Geometry check sheet. Reference: the model listing, model coordinates, mm. A direction names the side the tool comes from. Give positions to 0.01 mm unless a question says otherwise; leave off trailing zeros. Write each loop counter-clockwise with the first axis right and the second up, starting at its lowest first coordinate (ties: lowest second). Pieces come first, ordered by that corner, then holes. Notation, with made-up numbers: (12, 6) - (16, 6) arc R6 cw to (16, 15) - close; hole circle Ø3 at (20.5, -22.5). An arc over 180 degrees is marked (long way). Write item = value, one per line. Start each with the question number.
(1) Access from +Z, -Z, +X, -X, +Y, -Y to the whole of each face (thin tool, end or side, straight path). Record for faces 4 (the cylindrical face through (23.059, 0.513, 5.07)), 5 (the flat face through (21, 3, 3)), 6 (the cylindrical face through (18.541, 3.487, 5.07)).
(2) Section check B-B, the plane x = 17. Enter the section's corners in (y, z), plus the area to 3 significant figures.
(3) Depth check by flat-ended pin: pin 1 Ø1.5 at (y, z) = (3.5, 2) entering from +X; pin 2 Ø1.2 at (x, y) = (15.5, 2.5) entering from +Z; pin 3 Ø1 at (x, z) = (41.5, 2.5) entering from -Y. Enter the tip coordinate at first touch or a pass-through.
(4) Draft check along Y on faces 1 (the flat face through (57, 3, 3)), 2 (the cylindrical face through (68.059, 0.513, 3.221)), 3 (the flat face through (61, 2, 0)). Enter one of: pulls with the +Y half, pulls with the -Y half, needs draft (parallel to the pull), parting line crosses it, or undercut.
(5) Section check A-A, the plane z = 1. Give the number of separate pieces and of enclosed holes in the cut face, plus the area to 4 significant figures.
(6) Thickness scan on L1, parallel to Y at x = 12, z = 0.5; L2, parallel to Z at x = 36, y = 3.2; L3, parallel to X at y = 3.65, z = -3. Record the ranges inside material, lowest first.
```python
from build123d import *

# Parameters (mm, degrees)
SKETCH008_W     = 68.6
SKETCH008_H     = 4
PAD_DEPTH       = 3.75
SKETCH_W        = 5.6
SKETCH_H        = 4
PAD001_DEPTH    = 10
SKETCH001_W     = 5.6
SKETCH001_H     = 4
PAD002_DEPTH    = 10
SKETCH002_W     = 5.6
SKETCH002_H     = 4
PAD003_DEPTH    = 10
SKETCH003_W     = 5.6
SKETCH003_H     = 4
PAD004_DEPTH    = 10
SKETCH004_W     = 5.6
SKETCH004_H     = 4
PAD005_DEPTH    = 10
SKETCH005_W     = 5.6
SKETCH005_H     = 4
PAD006_DEPTH    = 10
SKETCH006_W     = 5.6
SKETCH006_H     = 4
PAD007_DEPTH    = 10
SKETCH007_W     = 5.6
SKETCH007_H     = 4
PAD008_DEPTH    = 10
SKETCH009_W     = 3.6
SKETCH009_H     = 2
POCKET_DEPTH    = 13.75
SKETCH010_W     = 3.6
SKETCH010_H     = 2
POCKET001_DEPTH = 13.75
SKETCH011_W     = 3.6
SKETCH011_H     = 2
POCKET002_DEPTH = 13.75
SKETCH012_W     = 3.6
SKETCH012_H     = 2
POCKET003_DEPTH = 13.75
SKETCH013_W     = 3.6
SKETCH013_H     = 2
POCKET004_DEPTH = 13.75
SKETCH014_W     = 3.6
SKETCH014_H     = 2
POCKET005_DEPTH = 13.75
SKETCH015_W     = 3.6
SKETCH015_H     = 2
POCKET006_DEPTH = 13.75
SKETCH016_W     = 3.6
SKETCH016_H     = 2
POCKET007_DEPTH = 13.75
FILLET_R        = 1.8


with BuildPart() as part:
    # Sketch008 → Pad (new body)
    with BuildSketch(Plane.XY):
        with Locations((34.3, 2)):
            Rectangle(SKETCH008_W, SKETCH008_H)
    extrude(amount=-PAD_DEPTH)

    # Sketch → Pad001 (join)
    with BuildSketch(Plane.XY):
        with Locations((2.8, 2)):
            Rectangle(SKETCH_W, SKETCH_H)
    extrude(amount=PAD001_DEPTH)

    # Sketch001 → Pad002 (join)
    with BuildSketch(Plane.XY):
        with Locations((11.8, 2)):
            Rectangle(SKETCH001_W, SKETCH001_H)
    extrude(amount=PAD002_DEPTH)

    # Sketch002 → Pad003 (join)
    with BuildSketch(Plane.XY):
        with Locations((20.8, 2)):
            Rectangle(SKETCH002_W, SKETCH002_H)
    extrude(amount=PAD003_DEPTH)

    # Sketch003 → Pad004 (join)
    with BuildSketch(Plane.XY):
        with Locations((29.8, 2)):
            Rectangle(SKETCH003_W, SKETCH003_H)
    extrude(amount=PAD004_DEPTH)

    # Sketch004 → Pad005 (join)
    with BuildSketch(Plane.XY):
        with Locations((38.8, 2)):
            Rectangle(SKETCH004_W, SKETCH004_H)
    extrude(amount=PAD005_DEPTH)

    # Sketch005 → Pad006 (join)
    with BuildSketch(Plane.XY):
        with Locations((47.8, 2)):
            Rectangle(SKETCH005_W, SKETCH005_H)
    extrude(amount=PAD006_DEPTH)

    # Sketch006 → Pad007 (join)
    with BuildSketch(Plane.XY):
        with Locations((56.8, 2)):
            Rectangle(SKETCH006_W, SKETCH006_H)
    extrude(amount=PAD007_DEPTH)

    # Sketch007 → Pad008 (join)
    with BuildSketch(Plane.XY):
        with Locations((65.8, 2)):
            Rectangle(SKETCH007_W, SKETCH007_H)
    extrude(amount=PAD008_DEPTH)

    # Sketch009 (on Face24 of Pad008) → Pocket (cut)
    with BuildSketch(Plane.XY.offset(10)):
        with Locations((2.8, 2)):
            Rectangle(SKETCH009_W, SKETCH009_H)
    extrude(amount=-POCKET_DEPTH, mode=Mode.SUBTRACT)

    # Sketch010 (on Face27 of Pad008) → Pocket001 (cut)
    with BuildSketch(Plane.XY.offset(10)):
        with Locations((11.8, 2)):
            Rectangle(SKETCH010_W, SKETCH010_H)
    extrude(amount=-POCKET001_DEPTH, mode=Mode.SUBTRACT)

    # Sketch011 (on Face30 of Pad008) → Pocket002 (cut)
    with BuildSketch(Plane.XY.offset(10)):
        with Locations((20.8, 2)):
            Rectangle(SKETCH011_W, SKETCH011_H)
    extrude(amount=-POCKET002_DEPTH, mode=Mode.SUBTRACT)

    # Sketch012 (on Face33 of Pad008) → Pocket003 (cut)
    with BuildSketch(Plane.XY.offset(10)):
        with Locations((29.8, 2)):
            Rectangle(SKETCH012_W, SKETCH012_H)
    extrude(amount=-POCKET003_DEPTH, mode=Mode.SUBTRACT)

    # Sketch013 (on Face36 of Pad008) → Pocket004 (cut)
    with BuildSketch(Plane.XY.offset(10)):
        with Locations((38.8, 2)):
            Rectangle(SKETCH013_W, SKETCH013_H)
    extrude(amount=-POCKET004_DEPTH, mode=Mode.SUBTRACT)

    # Sketch014 (on Face39 of Pad008) → Pocket005 (cut)
    with BuildSketch(Plane.XY.offset(10)):
        with Locations((47.8, 2)):
            Rectangle(SKETCH014_W, SKETCH014_H)
    extrude(amount=-POCKET005_DEPTH, mode=Mode.SUBTRACT)

    # Sketch015 (on Face42 of Pad008) → Pocket006 (cut)
    with BuildSketch(Plane.XY.offset(10)):
        with Locations((56.8, 2)):
            Rectangle(SKETCH015_W, SKETCH015_H)
    extrude(amount=-POCKET006_DEPTH, mode=Mode.SUBTRACT)

    # Sketch016 (on Face44 of Pad008) → Pocket007 (cut)
    with BuildSketch(Plane.XY.offset(10)):
        with Locations((65.8, 2)):
            Rectangle(SKETCH016_W, SKETCH016_H)
    extrude(amount=-POCKET007_DEPTH, mode=Mode.SUBTRACT)

    # Fillet
    fillet_edges = [part.edges().sort_by_distance(p)[0] for p in [
        (0, 4, 5),
        (0, 0, 5),
        (5.6, 4, 5),
        (5.6, 0, 5),
        (9, 0, 5),
        (9, 4, 5),
        (14.6, 4, 5),
        (14.6, 0, 5),
        (18, 4, 5),
        (18, 0, 5),
        (23.6, 4, 5),
        (23.6, 0, 5),
        (27, 4, 5),
        (27, 0, 5),
        (32.6, 4, 5),
        (32.6, 0, 5),
        (36, 4, 5),
        (41.6, 4, 5),
        (36, 0, 5),
        (41.6, 0, 5),
        (45, 4, 5),
        (45, 0, 5),
        (50.6, 0, 5),
        (50.6, 4, 5),
        (54, 4, 5),
        (59.6, 4, 5),
        (59.6, 0, 5),
        (54, 0, 5),
        (63, 4, 5),
        (63, 0, 5),
        (68.6, 0, 5),
        (68.6, 4, 5),
    ]]
    fillet(fillet_edges, radius=FILLET_R)


solid = part.part
```
Model answer:
q1.face_4 = +Z, -Y
q1.face_5 = +Z, -Z
q1.face_6 = +Z, +Y
q2.outline = (0, -3.75) - (4, -3.75) - (4, 0) - (0, 0) - close
q2.area = 15.0 mm²
q3.pin_1 = 68.51
q3.pin_2 = 0
q3.pin_3 = 0.46
q4.face_1 = undercut
q4.face_2 = pulls with the -Y half
q4.face_3 = needs draft
q5.separate_pieces = 8
q5.enclosed_holes = 8
q5.area = 99.35 mm²
q6.L1 = 0 to 1, 3 to 4
q6.L2 = -3.75 to 0
q6.L3 = 0.73 to 67.87
